from build123d import *
from build123d import SkipClean  # not in build123d's __all__

# Parameters (mm, degrees)
F1_R     = 41.5
F2_DEPTH = 1.5
F3_R     = 3.85
F4_DEPTH = 0.5
F6_DEPTH = 1.5


with BuildPart() as f2:
    # F1 (on face) → F2 (new body)
    with BuildSketch(Plane.XY):
        Circle(F1_R)
        with BuildLine():
            ThreePointArc((-28.8093051541, -27.7493051541), (-40, 0), (-28.8093051541, 27.7493051541))
            Line((-28.8093051541, 27.7493051541), (-20.0970856452, 19.0370856452))
            ThreePointArc((-20.0970856452, 19.0370856452), (-21.086593154, 15.6304460992), (-19.6150738914, 12.4026063935))
            ThreePointArc((-19.6150738914, 12.4026063935), (-18.9074615459, 12.1079784401), (-18.1991290923, 12.4008709077))
            Line((-18.1991290923, 12.4008709077), (-17.9308268662, 12.6691731338))
            Line((-17.9308268662, 12.6691731338), (-17.4883090065, 13.565932825))
            Line((-17.4883090065, 13.565932825), (-17.9010595127, 13.8481331433))
            Line((-17.9010595127, 13.8481331433), (-18.7223611076, 13.2776388924))
            ThreePointArc((-18.7223611076, 13.2776388924), (-18.7223611076, 18.7223611076), (-13.2776388924, 18.7223611076))
            Line((-13.2776388924, 18.7223611076), (-13.8477912725, 17.9008221471))
            Line((-13.8477912725, 17.9008221471), (-13.5657589526, 17.4879568294))
            Line((-13.5657589526, 17.4879568294), (-12.6691731338, 17.9308268662))
            Line((-12.6691731338, 17.9308268662), (-12.4008709077, 18.1991290923))
            ThreePointArc((-12.4008709077, 18.1991290923), (-12.1079784401, 18.9074615459), (-12.4026063935, 19.6150738914))
            ThreePointArc((-12.4026063935, 19.6150738914), (-15.6304460992, 21.086593154), (-19.0370856452, 20.0970856452))
            Line((-19.0370856452, 20.0970856452), (-27.7493051541, 28.8093051541))
            ThreePointArc((-27.7493051541, 28.8093051541), (0, 40), (27.7493051541, 28.8093051541))
            Line((27.7493051541, 28.8093051541), (19.0370856452, 20.0970856452))
            ThreePointArc((19.0370856452, 20.0970856452), (15.6304460992, 21.086593154), (12.4026063935, 19.6150738914))
            ThreePointArc((12.4026063935, 19.6150738914), (12.1079784401, 18.9074615459), (12.4008709077, 18.1991290923))
            Line((12.4008709077, 18.1991290923), (12.6691731338, 17.9308268662))
            Line((12.6691731338, 17.9308268662), (13.565932825, 17.4883090065))
            Line((13.565932825, 17.4883090065), (13.8481331433, 17.9010595127))
            Line((13.8481331433, 17.9010595127), (13.2776388924, 18.7223611076))
            ThreePointArc((13.2776388924, 18.7223611076), (18.7223611076, 18.7223611076), (18.7223611076, 13.2776388924))
            Line((18.7223611076, 13.2776388924), (17.9008221471, 13.8477912725))
            Line((17.9008221471, 13.8477912725), (17.4879568294, 13.5657589526))
            Line((17.4879568294, 13.5657589526), (17.9308268662, 12.6691731338))
            Line((17.9308268662, 12.6691731338), (18.1991290923, 12.4008709077))
            ThreePointArc((18.1991290923, 12.4008709077), (18.9074615459, 12.1079784401), (19.6150738914, 12.4026063935))
            ThreePointArc((19.6150738914, 12.4026063935), (21.086593154, 15.6304460992), (20.0970856452, 19.0370856452))
            Line((20.0970856452, 19.0370856452), (28.8093051541, 27.7493051541))
            ThreePointArc((28.8093051541, 27.7493051541), (40, 0), (28.8093051541, -27.7493051541))
            Line((28.8093051541, -27.7493051541), (20.0970856452, -19.0370856452))
            ThreePointArc((20.0970856452, -19.0370856452), (21.086593154, -15.6304460992), (19.6150738914, -12.4026063935))
            ThreePointArc((19.6150738914, -12.4026063935), (18.9074615459, -12.1079784401), (18.1991290923, -12.4008709077))
            Line((18.1991290923, -12.4008709077), (17.9308268662, -12.6691731338))
            Line((17.9308268662, -12.6691731338), (17.4883090065, -13.565932825))
            Line((17.4883090065, -13.565932825), (17.9010595127, -13.8481331433))
            Line((17.9010595127, -13.8481331433), (18.7223611076, -13.2776388924))
            ThreePointArc((18.7223611076, -13.2776388924), (18.7223611076, -18.7223611076), (13.2776388924, -18.7223611076))
            Line((13.2776388924, -18.7223611076), (13.8477912725, -17.9008221471))
            Line((13.8477912725, -17.9008221471), (13.5657589526, -17.4879568294))
            Line((13.5657589526, -17.4879568294), (12.6691731338, -17.9308268662))
            Line((12.6691731338, -17.9308268662), (12.4008709077, -18.1991290923))
            ThreePointArc((12.4008709077, -18.1991290923), (12.1079784401, -18.9074615459), (12.4026063935, -19.6150738914))
            ThreePointArc((12.4026063935, -19.6150738914), (15.6304460992, -21.086593154), (19.0370856452, -20.0970856452))
            Line((19.0370856452, -20.0970856452), (27.7493051541, -28.8093051541))
            ThreePointArc((27.7493051541, -28.8093051541), (0, -40), (-27.7493051541, -28.8093051541))
            Line((-27.7493051541, -28.8093051541), (-19.0370856452, -20.0970856452))
            ThreePointArc((-19.0370856452, -20.0970856452), (-15.6304460992, -21.086593154), (-12.4026063935, -19.6150738914))
            ThreePointArc((-12.4026063935, -19.6150738914), (-12.1079784401, -18.9074615459), (-12.4008709077, -18.1991290923))
            Line((-12.4008709077, -18.1991290923), (-12.6691731338, -17.9308268662))
            Line((-12.6691731338, -17.9308268662), (-13.565932825, -17.4883090065))
            Line((-13.565932825, -17.4883090065), (-13.8481331433, -17.9010595127))
            Line((-13.8481331433, -17.9010595127), (-13.2776388924, -18.7223611076))
            ThreePointArc((-13.2776388924, -18.7223611076), (-18.7223611076, -18.7223611076), (-18.7223611076, -13.2776388924))
            Line((-18.7223611076, -13.2776388924), (-17.9008221471, -13.8477912725))
            Line((-17.9008221471, -13.8477912725), (-17.4879568294, -13.5657589526))
            Line((-17.4879568294, -13.5657589526), (-17.9308268662, -12.6691731338))
            Line((-17.9308268662, -12.6691731338), (-18.1991290923, -12.4008709077))
            ThreePointArc((-18.1991290923, -12.4008709077), (-18.9074615459, -12.1079784401), (-19.6150738914, -12.4026063935))
            ThreePointArc((-19.6150738914, -12.4026063935), (-21.086593154, -15.6304460992), (-20.0970856452, -19.0370856452))
            Line((-20.0970856452, -19.0370856452), (-28.8093051541, -27.7493051541))
        make_face(mode=Mode.SUBTRACT)
    extrude(amount=F2_DEPTH)

    # F3 (on face) → F4 (cut)
    with BuildSketch(Plane.XY.offset(1.5)):
        with Locations((-16, 16)):
            Circle(F3_R)
        with Locations((-16, -16)):
            Circle(F3_R)
        with Locations((16, -16)):
            Circle(F3_R)
        with Locations((16, 16)):
            Circle(F3_R)
    with SkipClean():  # cleaning this boolean's faces spoils the solid; the shape is the same uncleaned
        extrude(amount=-F4_DEPTH, mode=Mode.SUBTRACT)

    # F5 (on Top) → F6 (join)
    with BuildSketch(Plane.XY):
        Polygon((-1.47, 41.4739568886), (-1.47, 43.4739568886), (-2.47, 43.4739568886), (-3.4575279787, 41.3557190758), align=None)
        Polygon((2.47, 43.4739568886), (1.47, 43.4739568886), (1.47, 41.4739568886), (3.4575279787, 41.3557190758), align=None)
        Polygon((-43.4739568886, 2.47), (-43.4739568886, 1.47), (-41.4739568886, 1.47), (-41.3557190758, 3.4575279787), align=None)
        Polygon((-41.4739568886, -1.47), (-43.4739568886, -1.47), (-43.4739568886, -2.47), (-41.3557190758, -3.4575279787), align=None)
        Polygon((-2.47, -43.4739568886), (-1.47, -43.4739568886), (-1.47, -41.4739568886), (-3.4575279787, -41.3557190758), align=None)
        Polygon((1.47, -41.4739568886), (1.47, -43.4739568886), (2.47, -43.4739568886), (3.4575279787, -41.3557190758), align=None)
        Polygon((43.4739568886, -2.47), (43.4739568886, -1.47), (41.4739568886, -1.47), (41.3557190758, -3.4575279787), align=None)
        Polygon((41.4739568886, 1.47), (43.4739568886, 1.47), (43.4739568886, 2.47), (41.3557190758, 3.4575279787), align=None)
    extrude(amount=F6_DEPTH)


solid = f2.part
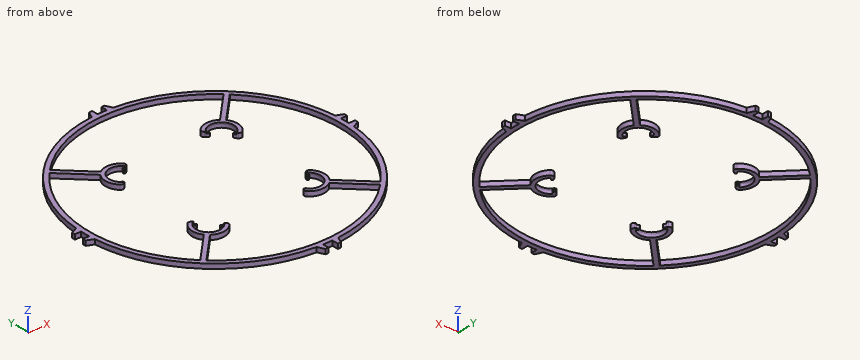
Geometry check sheet. Reference: the model listing, model coordinates, mm. Round coordinates to 2 decimals unless told otherwise and drop trailing zeros. Write each loop counter-clockwise with the first axis right and the second up, starting at its lowest first coordinate (ties: lowest second). Pieces come first, ordered by that corner, then holes. Notation, with made-up numbers: (-19, -2) - (3, -2) arc R21 cw to (3, 5) - close; hole circle Ø2 at (19, -18.75). An arc over 180 degrees is marked (long way). One line per item, written item: value.
1. Cross-section at C-C on y = -30. Record the boundary of the cut face in (x, z).
The answers:
outline: (-28.67, 0) - (-26.46, 0) - (-26.46, 1.5) - (-28.67, 1.5) - close; (26.46, 0) - (28.67, 0) - (28.67, 1.5) - (26.46, 1.5) - close
2. Cross-section at B-B on x = -16. Record the boundary of the cut face in (y, z).
The answers:
outline: (-38.29, 0) - (-36.66, 0) - (-36.66, 1.5) - (-38.29, 1.5) - close; (-21.1, 0) - (-19.85, 0) - (-19.85, 1.5) - (-21.1, 1.5) - close; (19.85, 0) - (21.1, 0) - (21.1, 1.5) - (19.85, 1.5) - close; (36.66, 0) - (38.29, 0) - (38.29, 1.5) - (36.66, 1.5) - close
3. Depth check by flat-ended pin: pin 1 Ø0.8 at (y, z) = (42, 0.5) entering from -X; pin 2 Ø0.8 at (x, z) = (-42.5, 0.5) entering from -Y; pin 3 Ø0.6 at (x, y) = (18, 13.5) entering from +Z. Enter the tip coordinate at first touch or a pass-through.
The answers:
pin 1: stops at x = -3.34
pin 2: stops at y = -3.11
pin 3: stops at z = 1
4. Scan lines: L1, parallel to X at y = 17, z = 0.6; L2, parallel to Y at x = -18, z = 0.65; L3, parallel to Y at x = 13.5, z = 1.45. Record each from-to range of solid material in increasing order.
The answers:
L1: x = -37.86 to -36.21, -21 to -19.72, 19.72 to 21, 36.21 to 37.86
L2: y = -37.39 to -35.72, -20.69 to -19.29, -13.78 to -12.6, 12.6 to 13.78, 19.29 to 20.69, 35.72 to 37.39
L3: y = -39.24 to -37.65, -20.45 to -18.93, 18.93 to 20.45, 37.65 to 39.24
5. Cross-section at A-A on x = 36. Record the boundary of the cut face in (y, z), and give its area (3 significant figures).
The answers:
outline: (-20.65, 0) - (-17.44, 0) - (-17.44, 1.5) - (-20.65, 1.5) - close; (17.44, 0) - (20.65, 0) - (20.65, 1.5) - (17.44, 1.5) - close
area: 9.63 mm^2
